from build123d import *

# Parameters (mm, degrees)
F0_W     = 161.877722
F0_H     = 103.971594
F1_DEPTH = 76.2
F2_R     = 15.793855
F3_DEPTH = 25.4
F4_R     = 11.063024
F5_DEPTH = 12.7


with BuildPart() as f1:
    # F0 (on Top) → F1 (new body)
    with BuildSketch(Plane.XY):
        Rectangle(F0_W, F0_H)
    extrude(amount=F1_DEPTH)

    # F2 (on face) → F3 (join)
    with BuildSketch(Plane.XY.offset(76.2)):
        with Locations((-51.472373, -20.210665)):
            Circle(F2_R)
    extrude(amount=F3_DEPTH)

    # F4 (on face) → F5 (cut, symmetric)
    with BuildSketch(Plane.XY.offset(101.6)):
        with Locations((-51.472373, -20.210665)):
            Circle(F4_R)
    extrude(amount=-F5_DEPTH, both=True, mode=Mode.SUBTRACT)


solid = f1.part
Here's how the part is built. I have some questions about the finished solid (model axes, mm). A direction names the side the tool comes from. Coordinates: 2 decimals unless noted, no trailing zeros. Write each loop counter-clockwise with the first axis right and the second up, starting at its lowest first coordinate (ties: lowest second). Pieces come first, ordered by that corner, then holes.
Item 1: Will these pins go through, and if not, where does the flat tip stop? pin 1 (1.5 mm diameter, centred on x = 16, y = 11, fed in from +Z); pin 2 (6.5 mm diameter, centred on x = -56.5, y = -19, fed in from +Z); pin 3 (4 mm diameter, centred on x = 25.5, y = 23.5, fed in from -Z).
Item 2: I want a section at C-C on x = 9.5. Write out the boundary of the cut face in (y, z).
Item 3: I want a section at B-B on z = 91.5. Write out the boundary of the cut face in (x, y), and give its area (3 significant figures).
Item 4: I want a section at A-A on y = -29. Write out the boundary of the cut face in (x, z).
Item 5: On a 3-axis mill with a long thin cutter (end or side, diameter ignored), from which of +Z, -Z, +X, -X, +Y, -Y can I reach the whole of each face in a straight line? I mean faces 5 (the flat face through (-1, -51.986, 38)), 6 (the cylindrical face through (-36.9, -26.3, 88.7)). Say none if no direction works.
Item 6: If we mould it in two halves opening along X, with no side actions, what happens to faces 1 (the flat face through (-1, 1, 0)), 2 (the flat face through (-52, -20, 88.9)), 3 (the flat face through (-80.939, -1, 38)), 4 (the cylindrical face through (-59.626, -12.734, 95.339))? For each: +X half, -X half, draft (parallel to the pull), parting line (faces both ways), or undercut.
Item 7: If I drill on line 1 (Z direction, x = 11, y = 30); line 2 (Y direction, x = -40.5, z = 85.5), over which ranges is the centre line in solid material (lowest first)?
Item 8: I want a section at D-D on y = -42.5. Write out the boundary of the cut face in (x, z).
Findings below:
1. pin 1: stops at z = 76.2
1. pin 2: stops at z = 88.9
1. pin 3: stops at z = 0
2. outline: (-51.99, 0) - (51.99, 0) - (51.99, 76.2) - (-51.99, 76.2) - close
3. outline: circle Ø31.59 at (-51.47, -20.21); hole circle Ø22.13 at (-51.47, -20.21)
3. area: 399 mm2
4. outline: (-80.94, 0) - (80.94, 0) - (80.94, 76.2) - (-38.35, 76.2) - (-38.35, 101.6) - (-44.75, 101.6) - (-44.75, 88.9) - (-58.19, 88.9) - (-58.19, 101.6) - (-64.59, 101.6) - (-64.59, 76.2) - (-80.94, 76.2) - close
5. face 5: +Z, -Z, +X, -X, -Y
5. face 6: +Z
6. face 1: draft
6. face 2: undercut
6. face 3: -X half
6. face 4: undercut
7. line 1: z = 0 to 76.2
7. line 2: y = -31.57 to -8.85
8. outline: (-80.94, 0) - (80.94, 0) - (80.94, 76.2) - (-80.94, 76.2) - close
